Here's how the part is built. I have some questions about the finished solid (model axes, mm). Coordinates: 2 decimals unless noted, no trailing zeros. Write each loop counter-clockwise with the first axis right and the second up, starting at its lowest first coordinate (ties: lowest second). Pieces come first, ordered by that corner, then holes. Notation, with made-up numbers: M -21.75,-30.5 L 36.25,-30.5 A12 cw 36.25,-21.5 Z; hole C 16,87.5 d4. An arc over 180 degrees is marked long. Use a Markdown table: item, result.
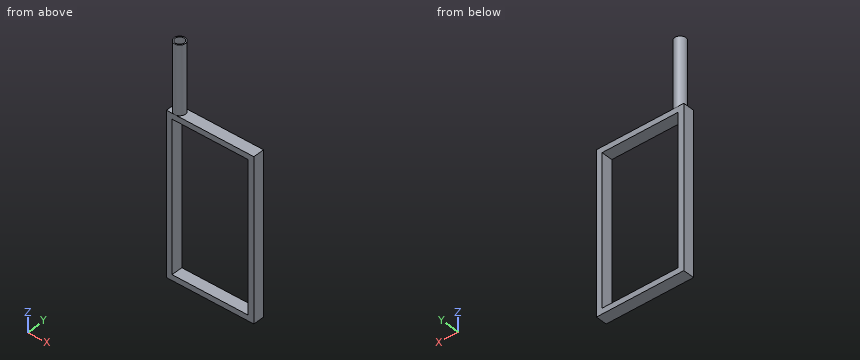
```python
from build123d import *

# Parameters (mm, degrees)
SCHIZZO1_W                   = 155
SCHIZZO1_H                   = 284
SCHIZZO1_W_2                 = 135
SCHIZZO1_H_2                 = 264
ESTRUSIONE_SOTTILE1_DEPTH    = 20
SCHIZZO2_R                   = 10
SCHIZZO2_R_2                 = 8
ESTRUSIONE_ESTRUSIONE1_DEPTH = 120


with BuildPart() as part:
    # Schizzo1 → Estrusione-Sottile1 (new body)
    with BuildSketch(Plane(origin=(0, 0, 0), x_dir=(1, 0, 0), z_dir=(0, 1, 0))):
        with Locations((67.5, 132)):
            Rectangle(SCHIZZO1_W, SCHIZZO1_H)
        with Locations((67.5, 132)):
            Rectangle(SCHIZZO1_W_2, SCHIZZO1_H_2, mode=Mode.SUBTRACT)
    extrude(amount=ESTRUSIONE_SOTTILE1_DEPTH)

    # Schizzo2 → Estrusione-Estrusione1 (add)
    with BuildSketch(Plane.XY.offset(10)):
        with Locations(Location((5, 10, 0), (0, 0, 270))):
            Circle(SCHIZZO2_R)
        with Locations((5, 10)):
            Circle(SCHIZZO2_R_2, mode=Mode.SUBTRACT)
    extrude(amount=ESTRUSIONE_ESTRUSIONE1_DEPTH)


solid = part.part
```
1. Will these pins go through, and if not, where does the flat tip stop? pin 1 Ø4.5 at (x, y) = (-1.5, 7.5) entering from +Z; pin 2 Ø10 at (x, y) = (49.5, 8.5) entering from +Z.
Answers follow:
| item | result |
|---|---|
| pin 1 | stops at z = 130 |
| pin 2 | stops at z = 10 |
2. I need wall thicknesses on probe 1 along Z at (x, y) = (110.5, 14); probe 2 along X at (y, z) = (10.25, -106); probe 3 along Z at (x, y) = (6, 1.5). Which ranges of each line are inside material? Lowest first, please.
Answers follow:
| item | result |
|---|---|
| probe 1 | z = -274 to -264, 0 to 10 |
| probe 2 | x = -10 to 0, 135 to 145 |
| probe 3 | z = -274 to -264, 0 to 130 |
3. Suppose I cut it at D-D on z = 22.5. Write out the boundary of the cut face in (x, y).
Answers follow:
| item | result |
|---|---|
| outline | C 5,10 d20; hole C 5,10 d16 |
4. Suppose I cut it at A-A on z = -53.5. Write out the boundary of the cut face in (x, y), and give its area (3 significant figures).
Answers follow:
| item | result |
|---|---|
| outline | M -10,0 L 0,0 L 0,20 L -10,20 Z; M 135,0 L 145,0 L 145,20 L 135,20 Z |
| area | 400 mm2 |
5. Suppose I cut it at B-B on x = 67.5. Write out the boundary of the cut face in (y, z), and give its area (3 significant figures).
Answers follow:
| item | result |
|---|---|
| outline | M 0,-274 L 20,-274 L 20,-264 L 0,-264 Z; M 0,0 L 20,0 L 20,10 L 0,10 Z |
| area | 400 mm2 |
6. Suppose I cut it at C-C on y = 10. Write out the boundary of the cut face in (x, z), and give its area (3 significant figures).
Answers follow:
| item | result |
|---|---|
| outline | M -10,-274 L 145,-274 L 145,10 L 15,10 L 15,130 L 13,130 L 13,10 L -3,10 L -3,130 L -5,130 L -5,10 L -10,10 Z; hole M 0,-264 L 135,-264 L 135,0 L 0,0 Z |
| area | 8,860 mm2 |
